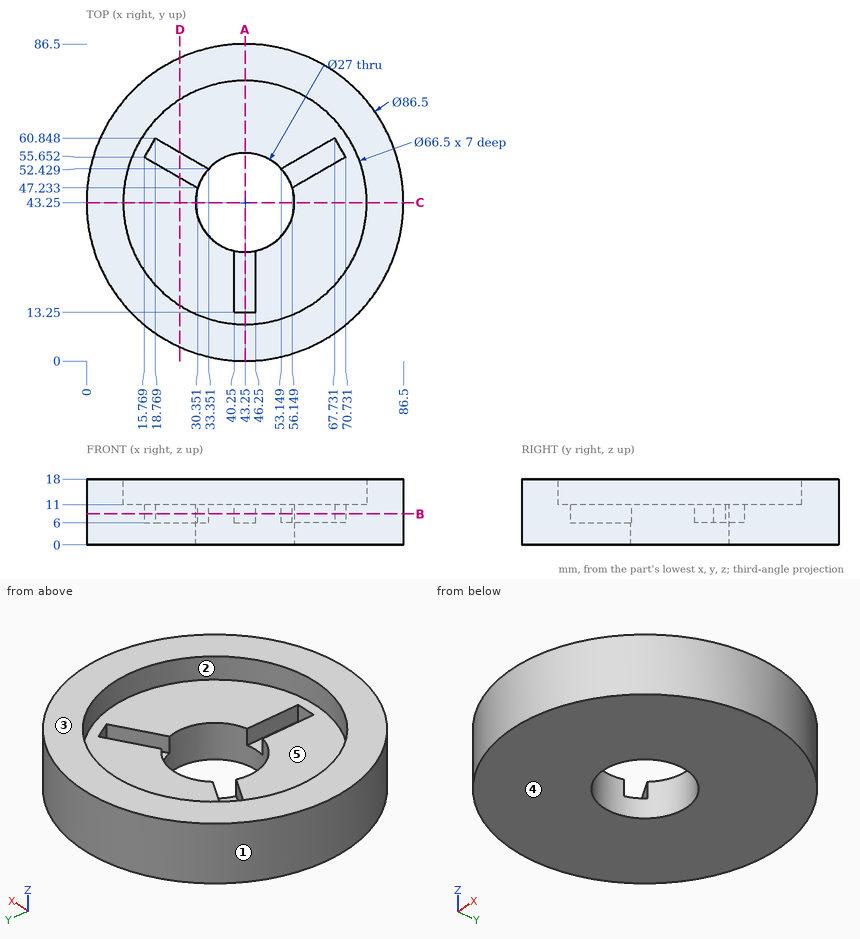
Input: dimensioned drawing with shaded views. Units: mm. Origin: part minimum x, y, z. A direction names the side the tool comes from. Coordinates: 2 decimals unless noted, no trailing zeros. Loops run counter-clockwise (first coordinate to the right, second up) from the corner with the lowest first, then second, coordinate; pieces in that order, holes last. Notation, with made-up numbers: (74, 73.5) -> (91, 73.5) arc R33 cw to (91, 102.5) -> close; hole circle Ø6 at (71.25, 88). An arc over 180 degrees is marked (long way). Use a Markdown table: item, result. Add a question column.
(1) Line query: line 1 along Y through (x, z) = (43.25, 15.75); line 2 along Z through (x, y) = (34, 56); line 3 along X through (y, z) = (26, 7.5). Output: solid intervals per line, ascending.
(2) Section query A-A, the plane x = 43.25. Return loops of the section in (y, z).
(3) Section query C-C, the plane y = 43.25. Return loops of the section in (x, z).
(4) Section query B-B, the plane z = 8.5. Return loops of the section in (x, y).
(5) Mould query, pull axis Y, two halves, no side actions, for the marked faces 1, 2 and 3. Classes: pulls with the +Y half, pulls with the -Y half, needs draft (parallel to the pull), parting line crosses it, or undercut.
(6) Access query for the marked faces 4 and 5. Directions: +Z, -Z, +X, -X, +Y, -Y. A direction counts if a zero-diameter tool reaches every point of the face in a straight line with its end or side. Return the directions, or none.
(7) Section query D-D, the plane x = 25.5. Return loops of the section in (y, z).
(8) Pin query (flat end, axial travel): pin 1 Ø4 at (y, z) = (24.5, 8) entering from +X (1 decimal); pin 2 Ø4 at (x, z) = (63.5, 2) entering from +Y; pin 3 Ø1 at (y, z) = (30.5, 16) entering from +X. Return the tip coordinate at first contact, or that it passes through.
Answer:
| question | item | result |
|---|---|---|
| 1 | line 1 | y = 0 to 10, 76.5 to 86.5 |
| 1 | line 2 | z = 0 to 11 |
| 1 | line 3 | x = 3.59 to 40.25, 46.25 to 82.91 |
| 2 | outline | (0, 0) -> (29.75, 0) -> (29.75, 6) -> (13.25, 6) -> (13.25, 11) -> (10, 11) -> (10, 18) -> (0, 18) -> close; (56.75, 0) -> (86.5, 0) -> (86.5, 18) -> (76.5, 18) -> (76.5, 11) -> (56.75, 11) -> close |
| 3 | outline | (0, 0) -> (29.75, 0) -> (29.75, 11) -> (10, 11) -> (10, 18) -> (0, 18) -> close; (56.75, 0) -> (86.5, 0) -> (86.5, 18) -> (76.5, 18) -> (76.5, 11) -> (56.75, 11) -> close |
| 4 | outline | circle Ø86.5 at (43.25, 43.25); hole (15.77, 55.65) -> (30.35, 47.23) arc R13.5 ccw to (40.25, 30.09) -> (40.25, 13.25) -> (46.25, 13.25) -> (46.25, 30.09) arc R13.5 ccw to (56.15, 47.23) -> (70.73, 55.65) -> (67.73, 60.85) -> (53.15, 52.43) arc R13.5 ccw to (33.35, 52.43) -> (18.77, 60.85) -> close |
| 5 | face 1 | parting line crosses it |
| 5 | face 2 | undercut |
| 5 | face 3 | needs draft |
| 6 | face 4 | -Z, +X, -X, +Y, -Y |
| 6 | face 5 | +Z |
| 7 | outline | (3.81, 0) -> (82.69, 0) -> (82.69, 18) -> (71.37, 18) -> (71.37, 11) -> (56.96, 11) -> (56.96, 6) -> (50.03, 6) -> (50.03, 11) -> (15.13, 11) -> (15.13, 18) -> (3.81, 18) -> close |
| 8 | pin 1 | stops at x = 83.1 |
| 8 | pin 2 | stops at y = 82.46 |
| 8 | pin 3 | stops at x = 84.73 |
